```python
from build123d import *

# Parameters (mm, degrees)
SKETCH_1_R          = 1.5
EXTRUDE_2_DEPTH     = 3
CUT_EXTRUDE_1_DEPTH = 10
SKETCH_4_R          = 7.5
CUT_EXTRUDE_2_DEPTH = 10
SKETCH_5_R          = 1.5
CUT_EXTRUDE_3_DEPTH = 10


with BuildPart() as part:
    # 草图1 → 凸台-拉伸2 (new body)
    with BuildSketch(Plane(origin=(0, 0, 0), x_dir=(1, 0, 0), z_dir=(0, 1, 0))):
        with BuildLine():
            Line((-60, 70), (60, 70))
            ThreePointArc((60, 70), (130, 0), (60, -70))
            Line((60, -70), (-60, -70))
            ThreePointArc((-60, -70), (-130, 0), (-60, 70))
        make_face()
        with Locations((-122, 0)):
            Circle(SKETCH_1_R, mode=Mode.SUBTRACT)
        with Locations((122, 0)):
            Circle(SKETCH_1_R, mode=Mode.SUBTRACT)
        with Locations((-30, 60)):
            Circle(SKETCH_1_R, mode=Mode.SUBTRACT)
        with Locations((30, 60)):
            Circle(SKETCH_1_R, mode=Mode.SUBTRACT)
        with Locations((30, -60)):
            Circle(SKETCH_1_R, mode=Mode.SUBTRACT)
        with Locations((-30, -60)):
            Circle(SKETCH_1_R, mode=Mode.SUBTRACT)
    extrude(amount=EXTRUDE_2_DEPTH)

    # 草图3 → 切除-拉伸1 (cut)
    with BuildSketch(Plane(origin=(0, 3, 0), x_dir=(1, 0, 0), z_dir=(0, 1, 0))):
        with BuildLine():
            Line((-60, -70), (60, -70))
            ThreePointArc((60, -70), (130, 0), (60, 70))
            Line((60, 70), (-60, 70))
            ThreePointArc((-60, 70), (-130, 0), (-60, -70))
        make_face()
        with BuildLine():
            Line((-60, -66), (60, -66))
            ThreePointArc((60, -66), (126, 0), (60, 66))
            Line((60, 66), (-60, 66))
            ThreePointArc((-60, 66), (-126, 0), (-60, -66))
        make_face(mode=Mode.SUBTRACT)
    extrude(amount=-CUT_EXTRUDE_1_DEPTH, mode=Mode.SUBTRACT)

    # 草图4 → 切除-拉伸2 (cut)
    with BuildSketch(Plane(origin=(0, 3, 0), x_dir=(1, 0, 0), z_dir=(0, 1, 0))):
        with Locations((-106, 0)):
            Circle(SKETCH_4_R)
        with Locations((106, 0)):
            Circle(SKETCH_4_R)
        with Locations((0, 46)):
            Circle(SKETCH_4_R)
        with Locations((0, -46)):
            Circle(SKETCH_4_R)
        with Locations((-60, -46)):
            Circle(SKETCH_4_R)
        with Locations((60, -46)):
            Circle(SKETCH_4_R)
        with Locations((30, -46)):
            Circle(SKETCH_4_R)
        with Locations((-30, -46)):
            Circle(SKETCH_4_R)
        with Locations((-92.526911935, -32.526911935)):
            Circle(SKETCH_4_R)
        with Locations((60, 46)):
            Circle(SKETCH_4_R)
        with Locations((30, 46)):
            Circle(SKETCH_4_R)
        with Locations((-92.526911935, 32.526911935)):
            Circle(SKETCH_4_R)
        with Locations((-30, 46)):
            Circle(SKETCH_4_R)
        with Locations((-60, 46)):
            Circle(SKETCH_4_R)
        with Locations((92.526911935, -32.526911935)):
            Circle(SKETCH_4_R)
        with Locations((92.526911935, 32.526911935)):
            Circle(SKETCH_4_R)
    extrude(amount=-CUT_EXTRUDE_2_DEPTH, mode=Mode.SUBTRACT)

    # 草图5 → 切除-拉伸3 (cut)
    with BuildSketch(Plane(origin=(0, 3, 0), x_dir=(1, 0, 0), z_dir=(0, 1, 0))):
        with Locations((-60, 63.5)):
            Circle(SKETCH_5_R)
        with Locations((114.99261314, 31.75)):
            Circle(SKETCH_5_R)
        with Locations((0, 63.5)):
            Circle(SKETCH_5_R)
        with Locations((60, 63.5)):
            Circle(SKETCH_5_R)
        with Locations((91.75, 54.99261314)):
            Circle(SKETCH_5_R)
        with Locations((91.75, -54.99261314)):
            Circle(SKETCH_5_R)
        with Locations((114.99261314, -31.75)):
            Circle(SKETCH_5_R)
        with Locations((-91.75, -54.99261314)):
            Circle(SKETCH_5_R)
        with Locations((-114.99261314, -31.75)):
            Circle(SKETCH_5_R)
        with Locations((-91.75, 54.99261314)):
            Circle(SKETCH_5_R)
        with Locations((-114.99261314, 31.75)):
            Circle(SKETCH_5_R)
        with Locations((60, -63.5)):
            Circle(SKETCH_5_R)
        with Locations((0, -63.5)):
            Circle(SKETCH_5_R)
        with Locations((-60, -63.5)):
            Circle(SKETCH_5_R)
    extrude(amount=-CUT_EXTRUDE_3_DEPTH, mode=Mode.SUBTRACT)


solid = part.part
```
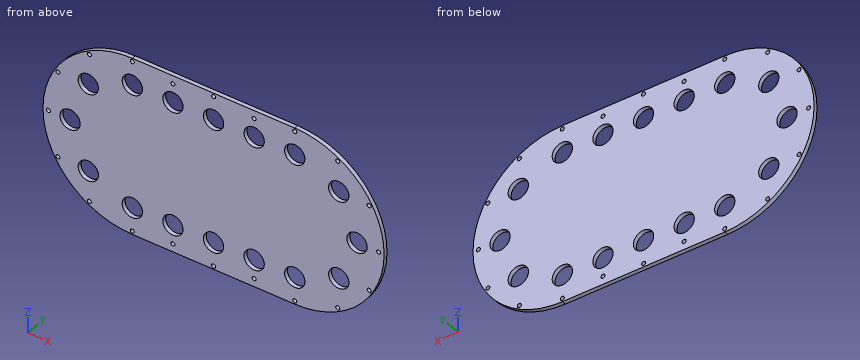
Geometry: final body of the model. Coordinates: model frame, mm. Round coordinates to 2 decimals unless told otherwise and drop trailing zeros. Loops run counter-clockwise (first coordinate to the right, second up) from the corner with the lowest first, then second, coordinate; pieces in that order, holes last. Notation, with made-up numbers: (28.25, 50) -> (76.25, 50) arc R27 cw to (76.25, 72) -> close; hole circle Ø5 at (73.25, 35.5). An arc over 180 degrees is marked (long way). Use one line per item in the form item = value. Start each with the question number.
1) Section C-C on z = -46. Output: boundary loops of the cut face in (x, y).
2) Section A-A on z = 4. Output: boundary loops of the cut face in (x, y).
3) Section B-B on x = 106. Output: boundary loops of the cut face in (y, z), then the cut area to 3 significant figures.
4) First-contact query: P1, Ø2.5, axis at x = -60, z = 63.5, coming from the +Y side. Flat tip, straight axial feed; report the tip coordinate or a pass-through.
5) Section D-D on y = 0.75. Give the number of separate pieces and of enclosed holes in the cut face, then the cut area to 3 significant figures.
6) Line query: L1, parallel to Z at x = 30, y = 1.1; L2, parallel to X at y = 1.9, z = 0; L3, parallel to Z at x = 86, y = 1.85. Output: solid intervals per line, ascending.
Response:
q1.outline = (-107.33, 0) -> (-67.5, 0) -> (-67.5, 3) -> (-107.33, 3) -> close; (-52.5, 0) -> (-37.5, 0) -> (-37.5, 3) -> (-52.5, 3) -> close; (-22.5, 0) -> (-7.5, 0) -> (-7.5, 3) -> (-22.5, 3) -> close; (7.5, 0) -> (22.5, 0) -> (22.5, 3) -> (7.5, 3) -> close; (37.5, 0) -> (52.5, 0) -> (52.5, 3) -> (37.5, 3) -> close; (67.5, 0) -> (107.33, 0) -> (107.33, 3) -> (67.5, 3) -> close
q2.outline = (-125.88, 0) -> (-112.34, 0) -> (-112.34, 3) -> (-125.88, 3) -> close; (-99.66, 0) -> (99.66, 0) -> (99.66, 3) -> (-99.66, 3) -> close; (112.34, 0) -> (125.88, 0) -> (125.88, 3) -> (112.34, 3) -> close
q3.outline = (0, -47.33) -> (3, -47.33) -> (3, -7.5) -> (0, -7.5) -> close; (0, 7.5) -> (3, 7.5) -> (3, 47.33) -> (0, 47.33) -> close
q3.area = 239 mm^2
q4.P1 = through
q5.separate_pieces = 1
q5.enclosed_holes = 36
q5.area = 26,600 mm^2
q6.L1 = -66 to -61.5, -58.5 to -53.5, -38.5 to 38.5, 53.5 to 58.5, 61.5 to 66
q6.L2 = -126 to -123.5, -120.5 to -113.5, -98.5 to 98.5, 113.5 to 120.5, 123.5 to 126
q6.L3 = -60.66 to -36.22, -28.83 to 28.83, 36.22 to 60.66
